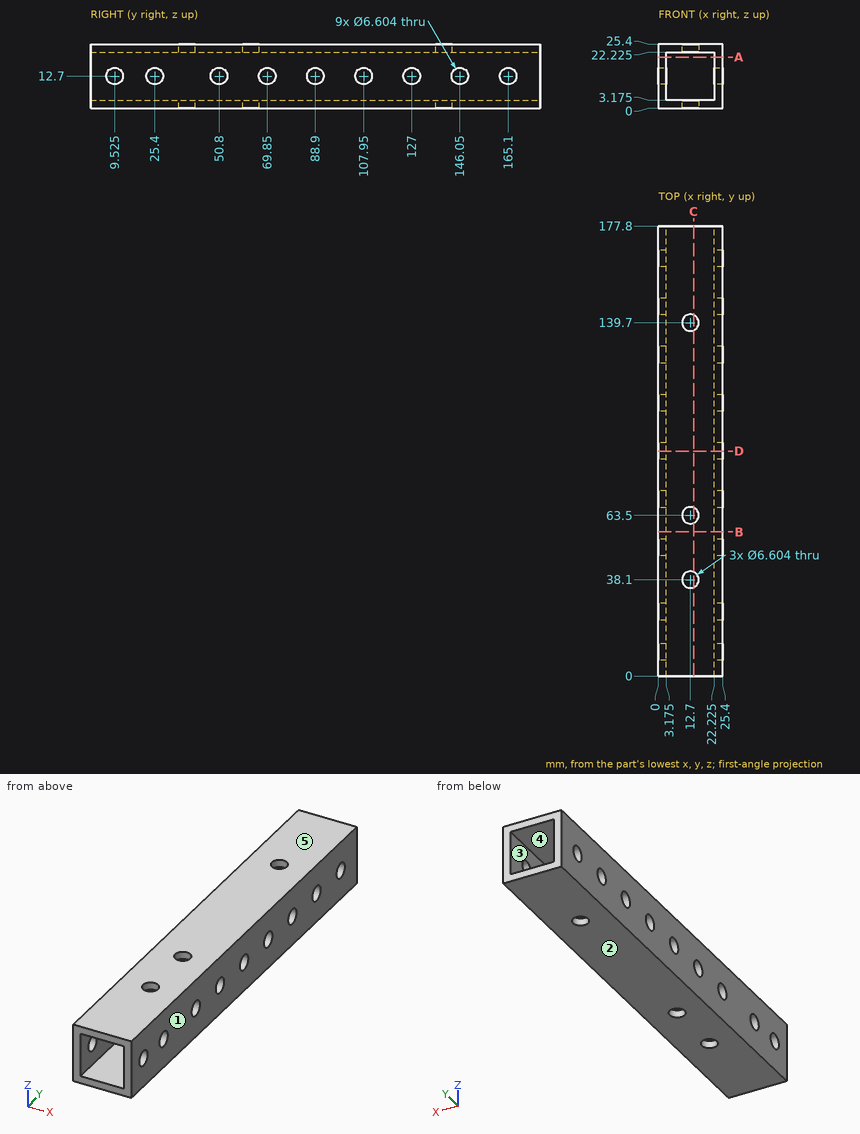
Here's the drawing with two shaded views (mm, measured from the low corner). I have some questions. A direction names the side the tool comes from. Coordinates: 2 decimals unless noted, no trailing zeros. Order: outer loops, then holes, each group sorted by start corner. A loop starts at its lowest first (then second) coordinate and runs counter-clockwise, first axis right, second up. Notation, with made-up numbers: M 25.5,-36.5 L 75.5,-36.5 A18 ccw 75.5,-7.5 Z; hole C -35.5,24.25 d3. An arc over 180 degrees is marked long. Answer as CSV lines item,"result".
Item 1: For pin 1 (4 mm diameter, centred on y = 69.85, z = 12.7, fed in from -X), with a flat end and sliding along its axis, tell me the tip position at first contact or that it passes through.
Results found:
pin 1,"through"
Item 2: On a 3-axis mill with a long thin cutter (end or side, diameter ignored), from which of +Z, -Z, +X, -X, +Y, -Y can I reach the whole of each face in a straight line? I mean the marked faces 4 and 5. Say none if no direction works.
Results found:
face 4,"+Y, -Y"
face 5,"+Z, +X, -X, +Y, -Y"
Item 3: Imagine slicing it at A-A on z = 20.25. Write out the boundary of the cut face in (x, y) (3 decimals), plus the area to 3 significant figures.
Results found:
outline,"M 0,0 L 3.175,0 L 3.175,177.8 L 0,177.8 Z; M 22.225,0 L 25.4,0 L 25.4,177.8 L 22.225,177.8 Z"
area,"1,130 mm2"
Item 4: We'd pull the mould along Z, two halves only. Please class the marked faces 1, 2 and 3: +Z half, -Z half, draft (parallel to the pull), parting line (faces both ways), or undercut.
Results found:
face 1,"draft"
face 2,"-Z half"
face 3,"undercut"
Item 5: Imagine slicing it at C-C on x = 14. Give the number of separate pieces and of enclosed holes in the cut face, plus the area to 3 significant figures.
Results found:
separate pieces,"8"
enclosed holes,"0"
area,"1,010 mm2"
Item 6: Imagine slicing it at B-B on y = 57. Write out the boundary of the cut face in (x, z) (3 decimals).
Results found:
outline,"M 0,0 L 25.4,0 L 25.4,25.4 L 0,25.4 Z; hole M 3.175,3.175 L 22.225,3.175 L 22.225,22.225 L 3.175,22.225 Z"
Item 7: Imagine slicing it at D-D on y = 88.9. Write out the boundary of the cut face in (x, z) (3 decimals), plus the area to 3 significant figures.
Results found:
outline,"M 0,0 L 25.4,0 L 25.4,9.398 L 22.225,9.398 L 22.225,3.175 L 3.175,3.175 L 3.175,9.398 L 0,9.398 Z; M 0,16.002 L 3.175,16.002 L 3.175,22.225 L 22.225,22.225 L 22.225,16.002 L 25.4,16.002 L 25.4,25.4 L 0,25.4 Z"
area,"240 mm2"
Item 8: If I drill on line 1 (Z direction, x = 12.5, y = 17.5) (3 decimals); line 2 (Y direction, x = 12.7, z = 1.15), over which ranges is the centre line in solid material (lowest first)?
Results found:
line 1,"0 to 3.175, 22.225 to 25.4"
line 2,"0 to 34.8, 41.4 to 60.2, 66.8 to 136.4, 143 to 177.8"
